Geometry check sheet. Reference: the model listing, model coordinates, mm. Coordinates: 2 decimals unless noted, no trailing zeros. Loops run counter-clockwise (first coordinate to the right, second up) from the corner with the lowest first, then second, coordinate; pieces in that order, holes last. Notation, with made-up numbers: (43, -23.75) -> (77, -23.75) arc R34 cw to (77, 14.25) -> close; hole circle Ø3 at (37.25, 57). An arc over 180 degrees is marked (long way). Answer as a JSON object with one key per item and string values.
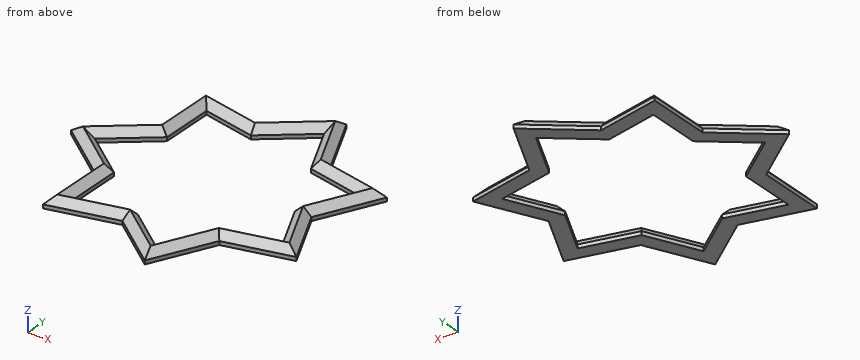
from build123d import *

# Parameters (mm, degrees)
F1_DEPTH = 3
F2_SIZE  = 1.99999


# Not quite as in the source:
# - a fillet or chamfer is up to 0.001 mm smaller than in the source, because OpenCascade refuses the exact size


with BuildPart() as f1:
    # F0 (on Top) → F1 (new body)
    with BuildSketch(Plane.XY):
        Polygon((6.0692586303, 20.150212978), (-2.1576516057, 37.2335681107), (-16.982031609, 25.4115195514), (-34.2207515071, 29.346144875), (-34.2207515071, 11.6640991742), (-48.8470692461, 0), (-34.2207515071, -11.6640991742), (-34.2207515071, -30.3718617382), (-15.982031609, -26.2089929403), (-1.6576516057, -37.6323048051), (6.2917795642, -21.1251408902), (24, -17.0833551327), (16.1191004999, -0.7184986964), (24.1784479339, 16.0169086929), align=None)
        Polygon((-42.4315673597, 0), (-30.2207515071, 9.737800699), (-30.2207515071, 24.3303035243), (-15.9941131941, 21.0831661669), (-3.5852350773, 30.9789162509), (3.3011727437, 16.6791430651), (18.3982804623, 13.2333267461), (11.6794354432, -0.7184986964), (18.2198325283, -14.2997731858), (3.5236936777, -17.6540709772), (-3.0852350773, -31.3776529454), (-14.9941131941, -21.8806395557), (-30.2207515071, -25.3560203876), (-30.2207515071, -9.737800699), align=None, mode=Mode.SUBTRACT)
    extrude(amount=F1_DEPTH)

    # F2 (size 2 in the source; OpenCascade refuses exactly that, so slightly less here)
    f2_edges = [f1.edges().sort_by_distance(p)[0] for p in [
        (15.123853, 18.083561, 3),
        (1.955804, 28.691891, 3),
        (-9.569842, 31.322544, 3),
        (-25.601392, 27.378832, 3),
        (-34.220752, 20.505122, 3),
        (-41.53391, 5.83205, 3),
        (-41.53391, -5.83205, 3),
        (-34.220752, -21.01798, 3),
        (-25.101392, -28.290427, 3),
        (-8.819842, -31.920649, 3),
        (2.317064, -29.378723, 3),
        (15.14589, -19.104248, 3),
        (20.05955, -8.900927, 3),
        (20.148774, 7.649205, 3),
        (-9.039674, -26.629146, 3),
        (-22.607432, -23.61833, 3),
        (-30.220752, -17.546911, 3),
        (-36.326159, -4.8689, 3),
        (-36.326159, 4.8689, 3),
        (-30.220752, 17.034052, 3),
        (-23.107432, 22.706735, 3),
        (-9.789674, 26.031041, 3),
        (-0.142031, 23.82903, 3),
        (10.849727, 14.956235, 3),
        (15.038858, 6.257414, 3),
        (14.949634, -7.509136, 3),
        (10.871763, -15.976922, 3),
        (0.219229, -24.515862, 3),
    ]]
    chamfer(f2_edges, length=F2_SIZE)


solid = f1.part
1. Section check B-B, the plane z = 0.55. Record the boundary of the cut face in (x, y), then the cut area to 3 significant figures.
Evaluation:
{"outline": "(-48.85, 0) -> (-34.22, -11.66) -> (-34.22, -30.37) -> (-15.98, -26.21) -> (-1.66, -37.63) -> (6.29, -21.13) -> (24, -17.08) -> (16.12, -0.72) -> (24.18, 16.02) -> (6.07, 20.15) -> (-2.16, 37.23) -> (-16.98, 25.41) -> (-34.22, 29.35) -> (-34.22, 11.66) -> close; hole (-42.43, 0) -> (-30.22, -9.74) -> (-30.22, -25.36) -> (-14.99, -21.88) -> (-3.09, -31.38) -> (3.52, -17.65) -> (18.22, -14.3) -> (11.68, -0.72) -> (18.4, 13.23) -> (3.3, 16.68) -> (-3.59, 30.98) -> (-15.99, 21.08) -> (-30.22, 24.33) -> (-30.22, 9.74) -> close", "area": "946 mm^2"}
2. Depth check by flat-ended pin: P1, Ø3, axis at x = 1.5, y = -19, coming from the +Z side; P2, Ø1.1, axis at y = 21, z = 0.5, coming from the -X side; P3, Ø1, axis at y = -13, z = 2.5, coming from the +X side. Enter the tip coordinate at first touch or a pass-through.
Evaluation:
{"P1": "stops at z = 1.26", "P2": "stops at x = -34.22", "P3": "stops at x = 20.97"}
3. Thickness scan on probe 1 along Y at (x, z) = (13.5, 1.9); probe 2 along Y at (x, z) = (18.5, 1.7); probe 3 along Y at (x, z) = (18, 1.7). Record the ranges inside material, lowest first. Write a range as from..to.
Evaluation:
{"probe 1": "y = -18.56..-16.3, -2.42..0.99, 15.27..17.53", "probe 2": "y = -17.62..-14.95, -13.27..-7.28, 5.84..11.83, 13.93..16.59", "probe 3": "y = -17.73..-15.07, -12.23..-6.24, 4.8..10.79, 14.04..16.71"}
